The listing builds one solid part. Answer for the finished solid, in the listing's coordinates (mm). Face numbers are marked on the shaded views. A direction names the side the tool comes from. Give positions to 0.01 mm unless a question says otherwise; leave off trailing zeros. Loops run counter-clockwise (first coordinate to the right, second up) from the corner with the lowest first, then second, coordinate; pieces in that order, holes last. Notation, with made-up numbers: M 80.5,70.25 L 111.5,70.25 A16 ccw 111.5,81.25 Z; hole C 57.5,-7.5 d11. An arc over 180 degrees is marked long. One line per item, written item: value. Start each with the question number.
Q1. The mould has two halves that part along X. Classify the marked faces 1, 2 and 3: +X half, -X half, draft (parallel to the pull), parting line (faces both ways), or undercut.
Q2. For the marked faces 4 and 5, determine the directions among +Z, -Z, +X, -X, +Y, -Y from which every point of the face is accessible in a straight line to the end or side of a thin tool.
Q3. Consider L1, parallel to X at y = 1.65, z = 0 (3 decimals); L2, parallel to X at y = 4.55, z = 0 (3 decimals); L3, parallel to Z at x = 5, y = 1.5. Determine where each line is inside the solid, lowest interval first.
Q4. A cutting plane is placed at A-A, the plane z = 0. Determine the outline of the cut face in (x, y) (3 decimals), and give its area (3 significant figures).
Q5. Flat-ended cylindrical pins translate along their axes: pin 1 (3 mm diameter, centred on y = 4.5, z = -8.5, fed in from -X); pin 2 (1.5 mm diameter, centred on x = -7.5, y = 4.5, fed in from +Z); pin 3 (2 mm diameter, centred on x = 4.5, z = -2, fed in from +Y). Find the tip coordinate at first contact, or state that the pin passes through.
from build123d import *

# Parameters (mm, degrees)
SKETCH1_R           = 16.51
SKETCH1_R_2         = 2.54
BOSS_EXTRUDE1_DEPTH = 6.35
SKETCH2_R           = 5.08
CUT_EXTRUDE1_DEPTH  = 3.81
FILLET1_R           = 1.27


with BuildPart() as part:
    # Sketch1 → Boss-Extrude1 (new body)
    with BuildSketch(Plane(origin=(0, 0, 0), x_dir=(1, 0, 0), z_dir=(0, 1, 0))):
        with Locations(Location((0, 0, 0), (0, 0, 270))):
            Circle(SKETCH1_R)
        with Locations(Location((-6.985, 0, 0), (0, 0, 270))):
            Circle(SKETCH1_R_2, mode=Mode.SUBTRACT)
        with Locations(Location((6.985, 0, 0), (0, 0, 90))):
            Circle(SKETCH1_R_2, mode=Mode.SUBTRACT)
    extrude(amount=BOSS_EXTRUDE1_DEPTH)

    # Sketch2 → Cut-Extrude1 (cut)
    with BuildSketch(Plane(origin=(0, 6.35, 0), x_dir=(1, 0, 0), z_dir=(0, 1, 0))):
        with Locations(Location((-6.985, 0, 0), (0, 0, 270))):
            Circle(SKETCH2_R)
        with Locations(Location((6.985, 0, 0), (0, 0, 270))):
            Circle(SKETCH2_R)
    extrude(amount=-CUT_EXTRUDE1_DEPTH, mode=Mode.SUBTRACT)

    # Fillet1
    fillet1_edges = [part.edges().sort_by_distance(p)[0] for p in [
        (0, 0, -16.51),
        (0, 6.35, -16.51),
    ]]
    fillet(fillet1_edges, radius=FILLET1_R)


solid = part.part
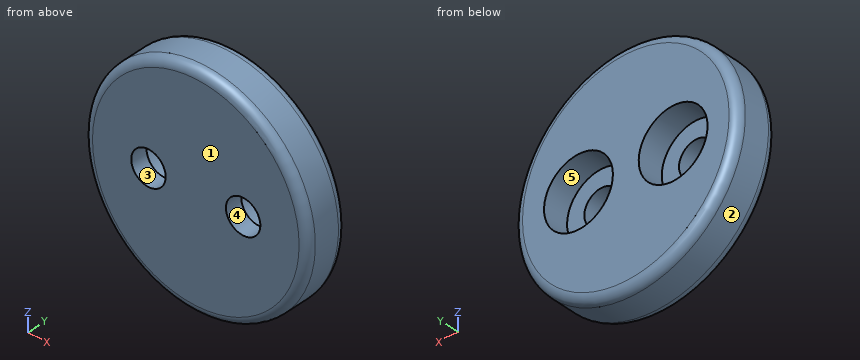
Answer block:
1. face 1: draft
1. face 2: parting line
1. face 3: undercut
2. face 4: +Y, -Y
2. face 5: +Y
3. L1: -16.51 to -9.525, -4.445 to 4.445, 9.525 to 16.51
3. L2: -16.51 to -12.065, -1.905 to 1.905, 12.065 to 16.51
3. L3: -15.73 to -1.58, 1.58 to 15.73
4. outline: M -16.51,1.27 A1.27 ccw -15.24,0 L -9.525,0 L -9.525,2.54 L -12.065,2.54 L -12.065,6.35 L -15.24,6.35 A1.27 ccw -16.51,5.08 Z; M -4.445,0 L 4.445,0 L 4.445,2.54 L 1.905,2.54 L 1.905,6.35 L -1.905,6.35 L -1.905,2.54 L -4.445,2.54 Z; M 9.525,0 L 15.24,0 A1.27 ccw 16.51,1.27 L 16.51,5.08 A1.27 ccw 15.24,6.35 L 12.065,6.35 L 12.065,2.54 L 9.525,2.54 Z
4. area: 105 mm^2
5. pin 1: x = -14.95
5. pin 2: z = 15.07
5. pin 3: y = 2.54
